Can you work these out from the model? Positions are in its coordinate system, mm. Face numbers are marked on the shaded views. A direction names the side the tool comes from. Round coordinates to 2 decimals unless told otherwise and drop trailing zeros. Loops run counter-clockwise (first coordinate to the right, second up) from the corner with the lowest first, then second, coordinate; pieces in that order, holes last. Notation, with made-up numbers: M 3.5,81.25 L 20.5,81.25 A23 cw 20.5,95.25 Z; hole C 63.5,-11.75 d3. An arc over 180 degrees is marked long. Use a Markdown table: item, result. Add a question column.
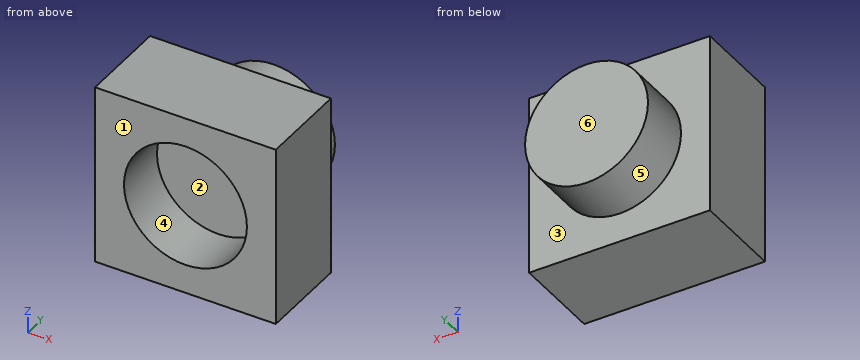
Autodesk Inventor part; units mm, degrees
ref_plane "YZ Plane" through (0, 0, 0) normal (1, 0, 0) x (0, 1, 0)
ref_plane "XZ Plane" through (0, 0, 0) normal (0, 1, 0) x (-1, 0, 0)
ref_plane "XY Plane" through (0, 0, 0) normal (0, 0, 1) x (1, 0, 0)
sketch "草圖1" plane through (0, 0, 0) normal (0, 1, 0) x (-1, 0, 0)
  line L0 (2.5, 2.5) -> (-2.5, 2.5)
  line L1 (-2.5, 2.5) -> (-2.5, -2.5)
  line L2 (-2.5, -2.5) -> (2.5, -2.5)
  line L3 (2.5, -2.5) -> (2.5, 2.5)
  circle A0 centre (0, 0) radius 1.7
  point P0 (2.5, 0)
  point P1 (0, -2.5)
  dimension "d0" = 5
  dimension "d1" = 5
  dimension "d4" = 3.4
extrude "擠出1" add sketch "草圖1" along normal blind 2.5 contours L3 L2 L1 L0 | A0
extrude "擠出2" cut sketch "草圖1" along normal blind 1.5 contours A0
sketch "草圖2" plane through (0, 2.5, 0) normal (0, 1, 0) x (1, 0, 0)
  circle A0 centre (0, 0) radius 1.7
extrude "擠出3" add sketch "草圖2" along normal blind 1.5
properties part number "110033226_ipt_06_磚塊樺木(1x1)"
(1) Thinking about a two-plate mould opening in X: for the marked faces 4, 5 and 6, which applies, released by +X, released by -X, zero draft, split by the parting line, or undercut?
(2) If I drill on probe 1 along Z at (x, y) = (0, 0.75); probe 2 along Y at (x, z) = (2.05, 1.6), over which ranges is the centre line in solid material (lowest first)? Write a range as [from, to].
(3) Suppose I cut it at C-C on x = 0. List the corners of the cut face in (y, z) for me, and give its area (3 significant figures).
(4) Suppose I cut it at B-B on z = 0. List the corners of the cut face in (x, y) for me.
(5) Suppose I cut it at A-A on y = 0.35. List the corners of the cut face in (x, z) for me.
(6) On a 3-axis mill with a long thin cutter (end or side, diameter ignored), from which of +Z, -Z, +X, -X, +Y, -Y can I reach the whole of each face in a straight line? I mean the marked faces 1, 2 and 3. Say none if no direction works.
Results below:
| question | item | result |
|---|---|---|
| 1 | face 4 | undercut |
| 1 | face 5 | split by the parting line |
| 1 | face 6 | zero draft |
| 2 | probe 1 | z = [-2.5, -1.7], [1.7, 2.5] |
| 2 | probe 2 | y = [0, 2.5] |
| 3 | outline | M 0,-2.5 L 2.5,-2.5 L 2.5,-1.7 L 4,-1.7 L 4,1.7 L 2.5,1.7 L 2.5,2.5 L 0,2.5 L 0,1.7 L 1.5,1.7 L 1.5,-1.7 L 0,-1.7 Z |
| 3 | area | 12.5 mm² |
| 4 | outline | M -2.5,0 L -1.7,0 L -1.7,1.5 L 1.7,1.5 L 1.7,0 L 2.5,0 L 2.5,2.5 L 1.7,2.5 L 1.7,4 L -1.7,4 L -1.7,2.5 L -2.5,2.5 Z |
| 5 | outline | M -2.5,-2.5 L 2.5,-2.5 L 2.5,2.5 L -2.5,2.5 Z; hole C 0,0 d3.4 |
| 6 | face 1 | +Z, -Z, +X, -X, -Y |
| 6 | face 2 | -Y |
| 6 | face 3 | +Y |
